Build history of the part. All positions in model axes, mm. Round coordinates to 2 decimals unless told otherwise and drop trailing zeros. Write each loop counter-clockwise with the first axis right and the second up, starting at its lowest first coordinate (ties: lowest second). Pieces come first, ordered by that corner, then holes.
1) Saw through at D-D (y = -35). Write the cut outline in (x, z), plus the area to 3 significant figures.
2) Saw through at C-C (x = -22). Write the cut outline in (y, z).
3) Flat gauge pins, fed straight in: pin 1 (2 mm diameter, centred on x = -65.22, y = -37.79, fed in from +Z); pin 2 (1 mm diameter, centred on y = -81.5, z = 3.5, fed in from +X); pin 3 (3 mm diameter, centred on y = -100, z = 2, fed in from +X). Where does each tip first touch, or does it go through?
4) Saw through at B-B (y = -73.5). Write the cut outline in (x, z).
5) Wall check: probe 1 along X at (y, z) = (-46, 1); probe 2 along X at (y, z) = (-62.5, 0.75); probe 3 along X at (y, z) = (-27, 3.6). Give the ranges that are in metal, low to high.
6) Saw through at A-A (z = 2.2). State how many separate pieces and enclosed holes the cut face has, plus the area to 3 significant figures.
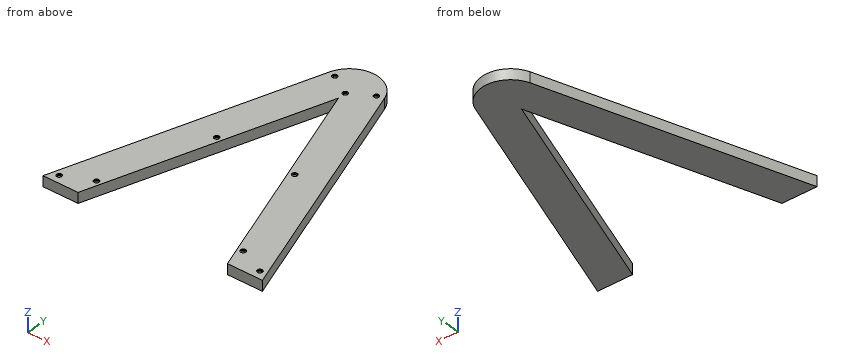
from build123d import *

# Parameters (mm, degrees)
F1_DEPTH = 5
F2_R     = 0.75
F3_DEPTH = 4.5
F4_R     = 1.25
F5_DEPTH = 0.5


with BuildPart() as f1:
    # F0 (on Top) → F1 (new body)
    with BuildSketch(Plane.XY):
        with BuildLine():
            Line((-101.1249, -149.980971), (-65.215021, -41.793592))
            Line((-65.215021, -41.793592), (-29.305143, -149.980971))
            Line((-29.305143, -149.980971), (-12.446784, -149.980971))
            Line((-12.446784, -149.980971), (-51.997887, -30.823505))
            ThreePointArc((-51.997887, -30.823505), (-65.215021, -21.439494), (-78.432156, -30.823505))
            Line((-78.432156, -30.823505), (-117.983259, -149.980971))
            Line((-117.983259, -149.980971), (-101.1249, -149.980971))
        make_face()
    extrude(amount=F1_DEPTH)

    # F2 (on face) → F3 (cut)
    with BuildSketch(Plane.XY.offset(5)):
        with Locations((-65.215021, -37.793592)):
            Circle(F2_R)
        with Locations((-113.483259, -145.980971)):
            Circle(F2_R)
        with Locations((-100.483259, -139.980971)):
            Circle(F2_R)
        with Locations((-29.946784, -139.980971)):
            Circle(F2_R)
        with Locations((-16.946784, -145.980971)):
            Circle(F2_R)
        with Locations((-83.983259, -89.980971)):
            Circle(F2_R)
        with Locations((-46.446784, -89.980971)):
            Circle(F2_R)
        with Locations((-75.215021, -31.793592)):
            Circle(F2_R)
        with Locations((-55.215021, -31.793592)):
            Circle(F2_R)
    extrude(amount=-F3_DEPTH, mode=Mode.SUBTRACT)

    # F4 (on face) → F5 (cut)
    with BuildSketch(Plane.XY.offset(5)):
        with Locations((-75.215021, -31.793592)):
            Circle(F4_R)
        with Locations((-65.215021, -37.793592)):
            Circle(F4_R)
        with Locations((-55.215021, -31.793592)):
            Circle(F4_R)
        with Locations((-46.446784, -89.980971)):
            Circle(F4_R)
        with Locations((-83.983259, -89.980971)):
            Circle(F4_R)
        with Locations((-16.946784, -145.980971)):
            Circle(F4_R)
        with Locations((-29.946784, -139.980971)):
            Circle(F4_R)
        with Locations((-100.483259, -139.980971)):
            Circle(F4_R)
        with Locations((-113.483259, -145.980971)):
            Circle(F4_R)
    extrude(amount=-F5_DEPTH, mode=Mode.SUBTRACT)


solid = f1.part
Evaluation:
1. outline: (-79.82, 0) - (-50.61, 0) - (-50.61, 5) - (-79.82, 5) - close
1. area: 146 mm2
2. outline: (-149.98, 0) - (-121.2, 0) - (-121.2, 5) - (-149.98, 5) - close
3. pin 1: stops at z = 4.5
3. pin 2: stops at x = -35.01
3. pin 3: stops at x = -28.54
4. outline: (-92.6, 0) - (-75.74, 0) - (-75.74, 5) - (-92.6, 5) - close; (-54.69, 0) - (-37.83, 0) - (-37.83, 5) - (-54.69, 5) - close
5. probe 1: x = -83.47 to -66.61, -63.82 to -46.96
5. probe 2: x = -88.95 to -72.09, -58.34 to -41.48
5. probe 3: x = -76.39 to -54.04
6. separate pieces: 1
6. enclosed holes: 9
6. area: 4,140 mm2
